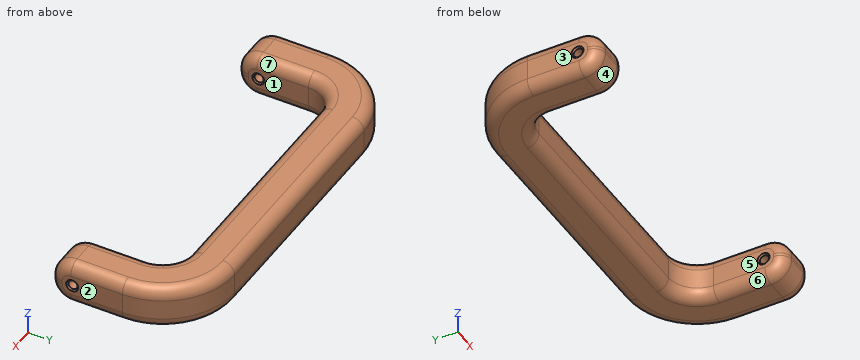
```python
from build123d import *

# Parameters (mm, degrees)
PAD_DEPTH    = 15
SKETCH001_R  = 1.6
POCKET_DEPTH = 130.001
FILLET_R     = 7
FILLET001_R  = 4
CHAMFER_SIZE = 0.5


with BuildPart() as part:
    # Sketch → Pad (new body)
    with BuildSketch(Plane.XY):
        with BuildLine():
            Line((-65, 0), (-65, 25))
            ThreePointArc((-40, 50), (-57.67767, 42.67767), (-65, 25))
            Line((-40, 50), (0, 50))
            Line((40, 50), (0, 50))
            ThreePointArc((65, 25), (57.67767, 42.67767), (40, 50))
            Line((65, 0), (65, 25))
            Line((65, 0), (50, 0))
            Line((50, 0), (50, 25))
            ThreePointArc((50, 25), (47.071068, 32.071068), (40, 35))
            Line((0, 35), (40, 35))
            Line((0, 35), (-40, 35))
            ThreePointArc((-40, 35), (-47.071068, 32.071068), (-50, 25))
            Line((-50, 0), (-50, 25))
            Line((-65, 0), (-50, 0))
        make_face()
    extrude(amount=PAD_DEPTH)

    # Sketch001 (on Face8 of Pad) → Pocket (cut, through all)
    with BuildSketch(Plane.YZ.offset(65)):
        with Locations((7.5, 7.5)):
            Circle(SKETCH001_R)
    extrude(amount=-POCKET_DEPTH, mode=Mode.SUBTRACT)

    # Fillet
    fillet_edges = [part.edges().sort_by_distance(p)[0] for p in [
        (57.5, 0, 0),
        (57.5, 0, 15),
        (-57.5, 0, 0),
        (-57.5, 0, 15),
    ]]
    fillet(fillet_edges, radius=FILLET_R)

    # Fillet001
    fillet001_edges = [part.edges().sort_by_distance(p)[0] for p in [
        (65, 2.050253, 12.949747),
        (0, 35, 0),
        (65, 0, 7.5),
        (65, 2.050253, 2.050253),
        (50, 2.050253, 2.050253),
        (50, 0, 7.5),
        (50, 2.050253, 12.949747),
        (50, 16, 15),
        (47.071068, 32.071068, 15),
        (65, 16, 15),
        (65, 16, 0),
        (57.67767, 42.67767, 15),
        (57.67767, 42.67767, 0),
        (0, 35, 15),
        (0, 50, 15),
        (-47.071068, 32.071068, 15),
        (-47.071068, 32.071068, 0),
        (-57.67767, 42.67767, 15),
        (-65, 16, 15),
        (-50, 16, 15),
        (-50, 2.050253, 12.949747),
        (-65, 2.050253, 12.949747),
        (-65, 0, 7.5),
        (-50, 0, 7.5),
        (-65, 2.050253, 2.050253),
        (-50, 2.050253, 2.050253),
        (-50, 16, 0),
        (-65, 16, 0),
        (-57.67767, 42.67767, 0),
        (0, 50, 0),
        (47.071068, 32.071068, 0),
        (50, 16, 0),
    ]]
    fillet(fillet001_edges, radius=FILLET001_R)

    # Chamfer
    chamfer_edges = [part.edges().sort_by_distance(p)[0] for p in [
        (-50, 5.9, 7.5),
        (65, 5.9, 7.5),
        (50, 5.9, 7.5),
        (-65, 5.9, 7.5),
    ]]
    chamfer(chamfer_edges, length=CHAMFER_SIZE)


solid = part.part
```
Geometry check sheet. Reference: the model listing, model coordinates, mm. Face numbers are marked on the shaded views. A direction names the side the tool comes from. Coordinates: 2 decimals unless noted, no trailing zeros. Order: outer loops, then holes, each group sorted by start corner. A loop starts at its lowest first (then second) coordinate and runs counter-clockwise, first axis right, second up. Notation, with made-up numbers: (84, -5.75) - (108, -5.75) arc R20 cw to (108, 20.25) - close; hole circle Ø4 at (47.25, 81). An arc over 180 degrees is marked (long way). Answer in a Markdown table with one row per item. Add a question column.
1. Section check B-B (x = 26). Enter the section's corners in (y, z).
2. Draft check along X on the marked faces 1, 2 and 3. Enter one of: +X half, -X half, draft (parallel to the pull), parting line (faces both ways), or undercut.
3. Section check A-A (y = 14.5). Enter the section's corners in (x, z), plus the area to 3 significant figures.
4. Gauge pin test, flat ends, axial feed: pin 1 Ø5 at (x, z) = (-48.5, 11) entering from +Y; pin 2 Ø4 at (y, z) = (9, 11.5) entering from +X; pin 3 Ø3.5 at (y, z) = (7.5, 7.5) entering from +X; pin 4 Ø3.5 at (y, z) = (7.5, 7.5) entering from -X. Record the tip position at first contact, or that the pin passes through.
5. Material ranges on L1, parallel to Z at x = 57, y = 7.5; L2, parallel to Y at x = -20.5, z = 5.25; L3, parallel to X at y = 32.5, z = 4, recorded low to high. Write a range as [from, to].
6. Access from +Z, -Z, +X, -X, +Y, -Y to the whole of each face (thin tool, end or side, straight path). Record for the marked faces 4, 5, 6 and 7.
Data:
| question | item | result |
|---|---|---|
| 1 | outline | (35, 4) arc R4 ccw to (39, 0) - (46, 0) arc R4 ccw to (50, 4) - (50, 11) arc R4 ccw to (46, 15) - (39, 15) arc R4 ccw to (35, 11) - close |
| 2 | face 1 | undercut |
| 2 | face 2 | +X half |
| 2 | face 3 | -X half |
| 3 | outline | (-65, 4) arc R4 ccw to (-61, 0) - (-54, 0) arc R4 ccw to (-50, 4) - (-50, 11) arc R4 ccw to (-54, 15) - (-61, 15) arc R4 ccw to (-65, 11) - close; (50, 4) arc R4 ccw to (54, 0) - (61, 0) arc R4 ccw to (65, 4) - (65, 11) arc R4 ccw to (61, 15) - (54, 15) arc R4 ccw to (50, 11) - close |
| 3 | area | 423 mm² |
| 4 | pin 1 | stops at y = 49.27 |
| 4 | pin 2 | stops at x = 65 |
| 4 | pin 3 | stops at x = 64.65 |
| 4 | pin 4 | stops at x = -64.65 |
| 5 | L1 | z = [0, 5.9], [9.1, 15] |
| 5 | L2 | y = [35, 50] |
| 5 | L3 | x = [-63.85, -46.61], [46.61, 63.85] |
| 6 | face 4 | -Z, +X, -X, -Y |
| 6 | face 5 | +Z, -Z, -Y |
| 6 | face 6 | -Z, -Y |
| 6 | face 7 | +Z, -Y |
